Design review of the part shown in the three views and the two pictorial views. Dimensions are in mm from the part's minimum x, y and z. A direction names the side the tool comes from. Give positions to 0.01 mm unless a question says otherwise; leave off trailing zeros. Order: outer loops, then holes, each group sorted by start corner. A loop starts at its lowest first (then second) coordinate and runs counter-clockwise, first axis right, second up. Notation, with made-up numbers: (-8.5, 29.25) - (0.5, 29.25) arc R29 ccw to (0.5, 65.25) - close; hole circle Ø9 at (45, 7). An arc over 180 degrees is marked (long way). Put each result on its own line as item: value.
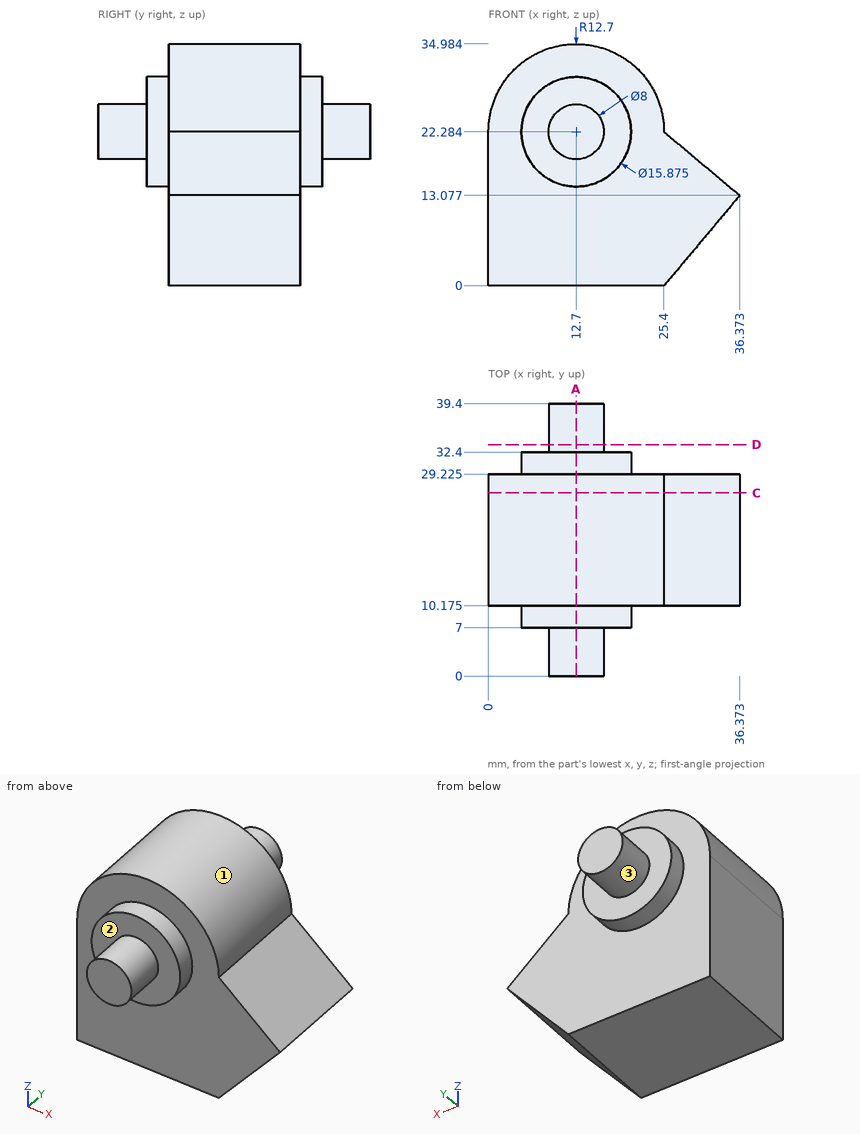
(1) Take a section at D-D, the plane y = 33.5. Write out the cut boundary in (x, z).
The answers:
outline: circle Ø8 at (12.7, 22.28)
(2) Wall thickness on L1, parallel to Y at x = 22, z = 11.5 (1 decimal); L2, parallel to X at y = 13.5, z = 9; L3, parallel to Z at x = 9.5, y = 38.5 (1 decimal): over which ranges is each line inside the solid? List them lowest first.
The answers:
L1: 10.2 to 29.2
L2: 0 to 32.95
L3: 19.9 to 24.7
(3) Take a section at C-C, the plane y = 26.5. Write out the cut boundary in (x, z), then the cut area to 3 significant figures.
The answers:
outline: (0, 0) - (25.4, 0) - (36.37, 13.08) - (25.4, 22.28) arc R12.7 ccw to (0, 22.28) - close
area: 942 mm^2
(4) Take a section at A-A, the plane x = 12.7. Write out the cut boundary in (y, z) (1 decimal), then the cut area to 3 significant figures.
The answers:
outline: (0, 18.3) - (7, 18.3) - (7, 14.3) - (10.2, 14.3) - (10.2, 0) - (29.2, 0) - (29.2, 14.3) - (32.4, 14.3) - (32.4, 18.3) - (39.4, 18.3) - (39.4, 26.3) - (32.4, 26.3) - (32.4, 30.2) - (29.2, 30.2) - (29.2, 35) - (10.2, 35) - (10.2, 30.2) - (7, 30.2) - (7, 26.3) - (0, 26.3) - close
area: 879 mm^2
(5) For the marked faces 1, 2 and 3, list the 3-axis set-ups (+Z, -Z, +X, -X, +Y, -Y) from which the entire face can be reached by the end or side of a thin tool; tool diameter is ignored.
The answers:
face 1: +Z, +Y, -Y
face 2: -Y
face 3: +Y
(6) Clearance check with flat-ended pins moving along their axes: pin 1 Ø5 at (y, z) = (11, 9) entering from +X; pin 2 Ø5 at (x, z) = (15, 8) entering from +Y (3 decimals); pin 3 Ø10.5 at (x, z) = (14, 11.5) entering from -Y. State where each tip first meets the part, or that it passes through.
The answers:
pin 1: x = 35.05
pin 2: y = 29.225
pin 3: y = 7
